For this review, take the finished solid that the model builds, in its own axes (mm). Coordinates: 2 decimals unless noted, no trailing zeros. Loops run counter-clockwise (first coordinate to the right, second up) from the corner with the lowest first, then second, coordinate; pieces in that order, holes last.
```python
from build123d import *

# Parameters (mm, degrees)
SKETCH1_R           = 1.778
BOSS_EXTRUDE1_DEPTH = 6.35


with BuildPart() as part:
    # Sketch1 → Boss-Extrude1 (new body)
    with BuildSketch(Plane.XZ):
        with BuildLine():
            Line((-58.674, -4.7625), (58.674, -4.7625))
            ThreePointArc((58.674, -4.7625), (63.4365, 0), (58.674, 4.7625))
            Line((58.674, 4.7625), (-58.674, 4.7625))
            ThreePointArc((-58.674, 4.7625), (-63.4365, 0), (-58.674, -4.7625))
        make_face()
        with Locations((58.674, 0)):
            Circle(SKETCH1_R, mode=Mode.SUBTRACT)
        with Locations((48.895, 0)):
            Circle(SKETCH1_R, mode=Mode.SUBTRACT)
        with Locations((39.116, 0)):
            Circle(SKETCH1_R, mode=Mode.SUBTRACT)
        with Locations((29.337, 0)):
            Circle(SKETCH1_R, mode=Mode.SUBTRACT)
        with Locations((19.558, 0)):
            Circle(SKETCH1_R, mode=Mode.SUBTRACT)
        with Locations((9.779, 0)):
            Circle(SKETCH1_R, mode=Mode.SUBTRACT)
        Circle(SKETCH1_R, mode=Mode.SUBTRACT)
        with Locations((-9.779, 0)):
            Circle(SKETCH1_R, mode=Mode.SUBTRACT)
        with Locations((-19.558, 0)):
            Circle(SKETCH1_R, mode=Mode.SUBTRACT)
        with Locations((-29.337, 0)):
            Circle(SKETCH1_R, mode=Mode.SUBTRACT)
        with Locations((-39.116, 0)):
            Circle(SKETCH1_R, mode=Mode.SUBTRACT)
        with Locations((-48.895, 0)):
            Circle(SKETCH1_R, mode=Mode.SUBTRACT)
        with Locations((-58.674, 0)):
            Circle(SKETCH1_R, mode=Mode.SUBTRACT)
    extrude(amount=-BOSS_EXTRUDE1_DEPTH)


solid = part.part
```
Q1. Wall thickness on probe 1 along Z at (x, y) = (-9.5, 0.75); probe 2 along Z at (x, y) = (40.5, 4); probe 3 along X at (y, z) = (5.5, 3.5): over which ranges is each line inside the solid? List them lowest first.
Q2. Consider section B-B (y = 4). Count the separate pieces of the cut face and the enclosed holes in it, then the cut area to 3 significant figures.
Q3. The part is to be moulded in two halves that separate along Z. For faces 1 (the face through (-57.03, 3.13, -0.68)), 2 (the face through (-1, 3, -4.762)), 3 (the face through (63.435, 3.131, -0.105)), 4 (the face through (-1, 0, 2)), say which applies: +Z half, -Z half, draft (parallel to the pull), parting line (faces both ways), or undercut.
Q4. Consider section A-A (x = 0). State the section outline as (y, z) points, then the cut area to 3 significant figures.
Model answer:
1. probe 1: z = -4.76 to -1.76, 1.76 to 4.76
1. probe 2: z = -4.76 to -1.12, 1.12 to 4.76
1. probe 3: x = -61.9 to 61.9
2. separate pieces: 1
2. enclosed holes: 13
2. area: 1,060 mm2
3. face 1: undercut
3. face 2: -Z half
3. face 3: parting line
3. face 4: draft
4. outline: (0, -4.76) - (6.35, -4.76) - (6.35, -1.78) - (0, -1.78) - close; (0, 1.78) - (6.35, 1.78) - (6.35, 4.76) - (0, 4.76) - close
4. area: 37.9 mm2
